Can you work these out from the model? Positions are in its coordinate system, mm. Face numbers are marked on the shaded views. A direction names the side the tool comes from. Give positions to 0.01 mm unless a question says otherwise; leave off trailing zeros. Loops run counter-clockwise (first coordinate to the right, second up) from the corner with the lowest first, then second, coordinate; pieces in that order, holes last. Notation, with made-up numbers: (-14, -10) - (4, -10) arc R24 ccw to (4, 1) - close; hole circle Ø4 at (32.25, 10.25). An arc over 180 degrees is marked (long way). Answer in a Markdown table with one row per item.
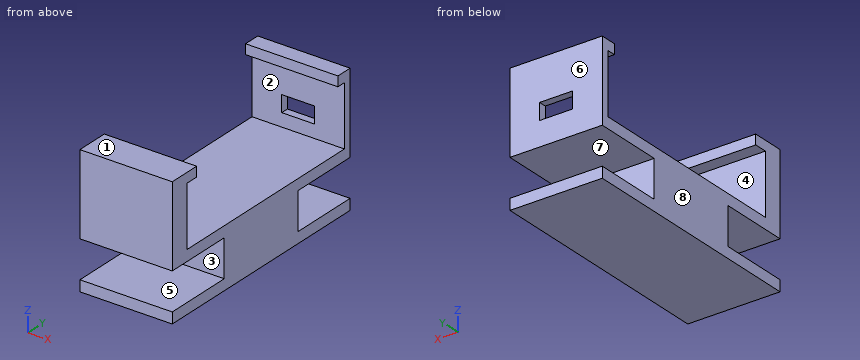
from build123d import *

# Parameters (mm, degrees)
F0_W      = 42
F0_H      = 109.5
F1_DEPTH  = 5
F2_W      = 42
F2_H      = 7.5
F2_H_2    = 15
F3_DEPTH  = 32
F4_W      = 42
F4_H      = 27.5
F5_DEPTH  = 4
F6_W      = 42
F6_H      = 27.5
F7_DEPTH  = 6
F8_W      = 15
F8_H      = 7.5
F9_DEPTH  = 3.501
F10_W     = 42
F10_H     = 54.75
F11_DEPTH = 22
F12_W     = 42
F12_H     = 17
F13_DEPTH = 32
F14_W     = 42
F14_H     = 17
F15_DEPTH = 32


# Not quite as in the source:
# - a feature names something its author has since deleted; it is built from what else it names


with BuildPart() as f1:
    # F0 (on Top) → F1 (new body)
    with BuildSketch(Plane.XY):
        Rectangle(F0_W, F0_H)
    extrude(amount=F1_DEPTH)

    # F2 (on face) → F3 (join)
    with BuildSketch(Plane.XY.offset(5)):
        with Locations((0, 51)):
            Rectangle(F2_W, F2_H)
        with Locations((0, -47.25)):
            Rectangle(F2_W, F2_H_2)
    extrude(amount=F3_DEPTH)

    # F4 (on face) → F5 (cut)
    with BuildSketch(Plane.XZ.offset(-47.25)):
        with Locations((0, 18.75)):
            Rectangle(F4_W, F4_H)
    extrude(amount=-F5_DEPTH, mode=Mode.SUBTRACT)

    # F6 (on face) → F7 (cut)
    with BuildSketch(Plane(origin=(0, -39.75, 0), x_dir=(-1, 0, 0), z_dir=(0, 1, 0))):
        with Locations((0, 18.75)):
            Rectangle(F6_W, F6_H)
    extrude(amount=-F7_DEPTH, mode=Mode.SUBTRACT)

    # F8 (on face) → F9 (cut, through all)
    with BuildSketch(Plane.XZ.offset(-51.25)):
        with Locations((0, 14.75)):
            Rectangle(F8_W, F8_H)
    extrude(amount=-F9_DEPTH, mode=Mode.SUBTRACT)

    # F10 (on face) → F11 (join)
    with BuildSketch(Plane(origin=(0, 0, 0), x_dir=(1, 0, 0), z_dir=(0, 0, -1))):
        with Locations((0, -27.375)):
            Rectangle(F10_W, F10_H)
        with Locations((0, 27.375)):
            Rectangle(F10_W, F10_H)
    extrude(amount=F11_DEPTH)

    # F12 (on face) → F13 (cut)
    with BuildSketch(Plane(origin=(0, 54.75, 0), x_dir=(-1, 0, 0), z_dir=(0, 1, 0))):
        with Locations((0, -8.5)):
            Rectangle(F12_W, F12_H)
    extrude(amount=-F13_DEPTH, mode=Mode.SUBTRACT)

    # F14 (on face) → F15 (cut)
    with BuildSketch(Plane.XZ.offset(54.75)):
        with Locations((0, -8.5)):
            Rectangle(F14_W, F14_H)
    extrude(amount=-F15_DEPTH, mode=Mode.SUBTRACT)


solid = f1.part
Q1. Imagine slicing it at C-C, the plane x = -5.5. Write out the boundary of the cut face in (y, z), and give its area (3 significant figures).
Checked values:
| item | result |
|---|---|
| outline | (-54.75, -22) - (54.75, -22) - (54.75, -17) - (22.75, -17) - (22.75, 0) - (54.75, 0) - (54.75, 11) - (51.25, 11) - (51.25, 5) - (-45.75, 5) - (-45.75, 32.5) - (-39.75, 32.5) - (-39.75, 37) - (-54.75, 37) - (-54.75, 0) - (-22.75, 0) - (-22.75, -17) - (-54.75, -17) - close; (47.25, 32.5) - (51.25, 32.5) - (51.25, 18.5) - (54.75, 18.5) - (54.75, 37) - (47.25, 37) - close |
| area | 2,290 mm² |
Q2. Imagine slicing it at B-B, the plane z = 9. Write out the boundary of the cut face in (x, y), and give its area (3 significant figures).
Checked values:
| item | result |
|---|---|
| outline | (-21, -54.75) - (21, -54.75) - (21, -45.75) - (-21, -45.75) - close; (-21, 51.25) - (21, 51.25) - (21, 54.75) - (-21, 54.75) - close |
| area | 525 mm² |
Q3. For pin 1 (8.5 mm diameter, centred on x = 1, z = -5, fed in from -Y); pin 2 (4 mm diameter, centred on x = 16, y = 14.5, fed in from +Z); pin 3 (4 mm diameter, centred on x = -3.5, z = 14, fed in from +Y), each with a flat end and sliding along its axis, tell me the tip position at first contact or that it passes through.
Checked values:
| item | result |
|---|---|
| pin 1 | stops at y = -22.75 |
| pin 2 | stops at z = 5 |
| pin 3 | stops at y = -45.75 |
Q4. Imagine slicing it at D-D, the plane x = -17.5. Write out the boundary of the cut face in (y, z), and give its area (3 significant figures).
Checked values:
| item | result |
|---|---|
| outline | (-54.75, -22) - (54.75, -22) - (54.75, -17) - (22.75, -17) - (22.75, 0) - (54.75, 0) - (54.75, 37) - (47.25, 37) - (47.25, 32.5) - (51.25, 32.5) - (51.25, 5) - (-45.75, 5) - (-45.75, 32.5) - (-39.75, 32.5) - (-39.75, 37) - (-54.75, 37) - (-54.75, 0) - (-22.75, 0) - (-22.75, -17) - (-54.75, -17) - close |
| area | 2,310 mm² |
Q5. If I drill on line 1 (Z direction, x = 0.5, y = -45); line 2 (Y direction, x = -19, z = 30); line 3 (Z direction, x = 6, y = 30.5), over which ranges is the centre line in solid material (lowest first)? Write a range as [from, to].
Checked values:
| item | result |
|---|---|
| line 1 | z = [-22, -17], [0, 5], [32.5, 37] |
| line 2 | y = [-54.75, -45.75], [51.25, 54.75] |
| line 3 | z = [-22, -17], [0, 5] |
Q6. If we mould it in two halves opening along Y, with no side actions, what happens to the marked faces 1, 2 and 3? For each: released by +Y, released by -Y, zero draft, split by the parting line, or undercut.
Checked values:
| item | result |
|---|---|
| face 1 | zero draft |
| face 2 | undercut |
| face 3 | released by -Y |
Q7. Imagine slicing it at A-A, the plane y = -47. Write out the boundary of the cut face in (x, z).
Checked values:
| item | result |
|---|---|
| outline | (-21, -22) - (21, -22) - (21, -17) - (-21, -17) - close; (-21, 0) - (21, 0) - (21, 37) - (-21, 37) - close |
Q8. On a 3-axis mill with a long thin cutter (end or side, diameter ignored), from which of +Z, -Z, +X, -X, +Y, -Y can I reach the whole of each face in a straight line? I mean the marked faces 4, 5, 6, 7 and 8. Say none if no direction works.
Checked values:
| item | result |
|---|---|
| face 4 | +X, -X |
| face 5 | +X, -X, -Y |
| face 6 | +Z, -Z, +X, -X, +Y |
| face 7 | +X, -X, +Y |
| face 8 | +Z, -Z, -X, +Y, -Y |
